Here's how the part is built. I have some questions about the finished solid (model axes, mm). Round coordinates to 2 decimals unless told otherwise and drop trailing zeros. Order: outer loops, then holes, each group sorted by start corner. A loop starts at its lowest first (then second) coordinate and runs counter-clockwise, first axis right, second up. Notation, with made-up numbers: (23, 41.5) - (40, 41.5) arc R21 ccw to (40, 71.5) - close; hole circle Ø4 at (44, -37). An arc over 180 degrees is marked (long way). Answer as a JSON object with one key per item and string values.
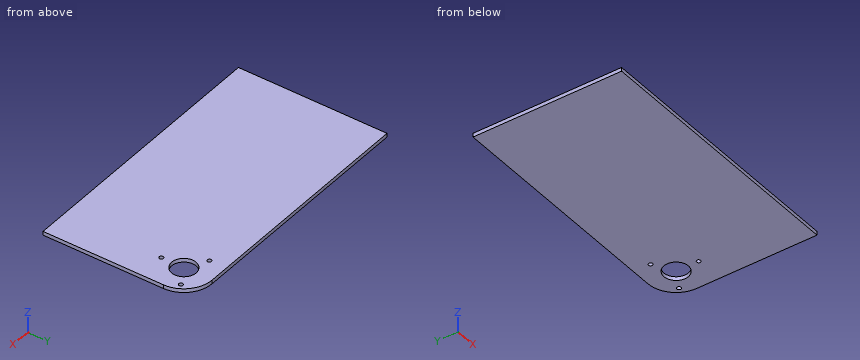
```python
from build123d import *

# Parameters (mm, degrees)
F0_W     = 226.934583
F0_H     = 125.4125
F0_R     = 1.7272
F0_R_2   = 10.31875
F1_DEPTH = 3.175
F2_R     = 23.8125


with BuildPart() as f1:
    # F0 (on Top) → F1 (new body)
    with BuildSketch(Plane.XY):
        with Locations((-113.467292, -62.70625)):
            Rectangle(F0_W, F0_H)
        with Locations((-23.8125, -42.8625)):
            Circle(F0_R, mode=Mode.SUBTRACT)
        with Locations((-23.8125, -23.8125)):
            Circle(F0_R_2, mode=Mode.SUBTRACT)
        with Locations((-40.310284, -14.2875)):
            Circle(F0_R, mode=Mode.SUBTRACT)
        with Locations((-7.314716, -14.2875)):
            Circle(F0_R, mode=Mode.SUBTRACT)
    extrude(amount=F1_DEPTH)

    # F2
    f2_edges = [f1.edges().sort_by_distance(p)[0] for p in [
        (0, 0, 1.5875),
    ]]
    fillet(f2_edges, radius=F2_R)


solid = f1.part
```
1. Imagine slicing it at A-A (y = -19). List the corners of the cut face in (x, z) for me (3 decimals), plus the area to 3 significant figures.
Responses:
{"outline": "(-226.935, 0) - (-32.94, 0) - (-32.94, 3.175) - (-226.935, 3.175) - close; (-14.685, 0) - (-0.491, 0) - (-0.491, 3.175) - (-14.685, 3.175) - close", "area": "661 mm2"}
2. If I drill on L1, parallel to Y at x = -28.5, z = 2.25; L2, parallel to Y at x = -17, z = 0.8; L3, parallel to X at y = -28, z = 2.4, over which ranges is the centre line in solid material (lowest first)? Write a range as [from, to].
Responses:
{"L1": "[-125.41, -33.01], [-14.62, 0]", "L2": "[-125.41, -31.56], [-16.06, -1]", "L3": "[-226.93, -33.24], [-14.38, 0]"}
3. Imagine slicing it at B-B (z = 0.7). List the corners of the cut face in (x, y) for me (1 decimal), plus the area to 3 significant figures.
Responses:
{"outline": "(-226.9, -125.4) - (0, -125.4) - (0, -23.8) arc R23.8 ccw to (-23.8, 0) - (-226.9, 0) - close; hole circle Ø3.5 at (-40.3, -14.3); hole circle Ø20.6 at (-23.8, -23.8); hole circle Ø3.5 at (-23.8, -42.9); hole circle Ø3.5 at (-7.3, -14.3)", "area": "28,000 mm2"}
